Could you check a few things on this model? Use its own coordinates, in mm. Coordinates: 2 decimals unless noted, no trailing zeros. Write each loop counter-clockwise with the first axis right and the second up, starting at its lowest first coordinate (ties: lowest second). Pieces come first, ordered by that corner, then holes. Notation, with made-up numbers: (5.5, 44) - (52.5, 44) arc R12 ccw to (52.5, 64) - close; hole circle Ø11 at (54.5, -3). An arc over 180 degrees is marked (long way). Answer as a JSON object with one key per item and string values. Group by question number.
1) We'd pull the mould along Y, two halves only. Please class faces 1 (the flat face through (48.138, -135.032, 1.565)), 2 (the flat face through (83, -127, 3.175)), 3 (the cylindrical face through (91.24, -191.55, 1.61)): released by +Y, released by -Y, zero draft, split by the parting line, or undercut.
2) Please list where these lines run through material, in increasing order: line 1 along X through (y, z) = (-172, 1.45); line 2 along X through (y, z) = (-19, 0.4).
3) If we section it at B-B (z = 2.1): Write out the boundary of the cut face in (x, y) (3 decimals).
4) If we section it at D-D (y = -84.5): Write out the boundary of the cut face in (x, z) (3 decimals).
5) If we section it at A-A (y = 0): Write out the boundary of the cut face in (x, z) (3 decimals), plus the area to 3 significant figures.
6) If we section it at C-C (x = 76.5): Write out the boundary of the cut face in (y, z) (3 decimals), plus the area to 3 significant figures.
```python
from build123d import *
from OCP.BRepFilletAPI import BRepFilletAPI_MakeFillet

# Parameters (mm, degrees)
SKETCH1_R           = 3.3
BOSS_EXTRUDE1_DEPTH = 3.175
FILLET1_R1          = 10
FILLET1_R2          = 3
SKETCH2_R           = 3.3
CUT_EXTRUDE1_DEPTH  = 312.546271304


with BuildPart() as part:
    # Sketch1 → Boss-Extrude1 (new body)
    with BuildSketch(Plane.XY):
        Polygon((72.5, 6.35), (167.244494596, -253.95835952), (97.244494596, -266.301248169), (0, -6.35), (0, 6.35), align=None)
        with Locations((53.975, 0)):
            Circle(SKETCH1_R, mode=Mode.SUBTRACT)
        with Locations((15.875, 0)):
            Circle(SKETCH1_R, mode=Mode.SUBTRACT)
    extrude(amount=BOSS_EXTRUDE1_DEPTH)

    # Fillet1: one fillet with a radius per group of edges: ONE call of the kernel's fillet builder (fillet() takes one radius for all edges)
    fillet1_edges_1 = [part.edges().sort_by_distance(p)[0] for p in [
        (167.244494596, -253.95835952, 1.5875),
        (97.244494596, -266.301248169, 1.5875),
        (0, -6.35, 1.5875),
    ]]
    fillet1_edges_2 = [part.edges().sort_by_distance(p)[0] for p in [
        (72.5, 6.35, 1.5875),
        (0, 6.35, 1.5875),
    ]]
    fillet1 = BRepFilletAPI_MakeFillet(part.part.solid().wrapped)
    for e in fillet1_edges_1:
        fillet1.Add(FILLET1_R1, e.wrapped)
    for e in fillet1_edges_2:
        fillet1.Add(FILLET1_R2, e.wrapped)
    add(Compound.cast(fillet1.Shape()), mode=Mode.REPLACE)

    # Sketch2 → Cut-Extrude1 (cut, through all)
    with BuildSketch(Plane.XY.offset(3.175)):
        with Locations((94.53593378, -191.691292203)):
            Circle(SKETCH2_R)
    extrude(amount=-CUT_EXTRUDE1_DEPTH, mode=Mode.SUBTRACT)


solid = part.part
```
Here are the results:
{
 "1": {"face 1": "released by -Y", "face 2": "zero draft", "face 3": "undercut"},
 "2": {"line 1": "x = 61.97 to 137.41", "line 2": "x = 4.73 to 81.73"},
 "3": {"outline": "(0, -4.541) arc R10 ccw to (0.634, -8.045) - (94.331, -258.513) arc R10 ccw to (105.434, -264.857) - (155.508, -256.028) arc R10 ccw to (163.168, -242.76) - (73.218, 4.376) arc R3 ccw to (70.399, 6.35) - (3, 6.35) arc R3 ccw to (0, 3.35) - close; hole circle Ø6.6 at (15.875, 0); hole circle Ø6.6 at (53.975, 0); hole circle Ø6.6 at (94.536, -191.691)"},
 "4": {"outline": "(29.235, 0) - (105.567, 0) - (105.567, 3.175) - (29.235, 3.175) - close"},
 "5": {"outline": "(0, 0) - (12.575, 0) - (12.575, 3.175) - (0, 3.175) - close; (19.175, 0) - (50.675, 0) - (50.675, 3.175) - (19.175, 3.175) - close; (57.275, 0) - (74.811, 0) - (74.811, 3.175) - (57.275, 3.175) - close", "area": "196 mm²"},
 "6": {"outline": "(-210.848, 0) - (-4.64, 0) - (-4.64, 3.175) - (-210.848, 3.175) - close", "area": "655 mm²"}
}
